Could you check a few things on this model? Use its own coordinates, in mm. Face numbers are marked on the shaded views. Give positions to 0.01 mm unless a question says otherwise; leave off trailing zeros. Loops run counter-clockwise (first coordinate to the right, second up) from the corner with the lowest first, then second, coordinate; pieces in that order, holes last. Notation, with made-up numbers: M 80.5,25.5 L 133.5,25.5 A31 cw 133.5,56.5 Z; hole C 2,74.5 d6. An arc over 180 degrees is marked long. Write each question's results on one line, items separated by ' | '. Start each with the question number.
from build123d import *

# Parameters (mm, degrees)
SKETCH1_W               = 10
SKETCH1_H               = 10
BOSS_EXTRUDE1_DEPTH     = 85
SKETCH2_W               = 10
SKETCH2_H               = 8.2
CUT_EXTRUDE1_DEPTH      = 2.5
CUT_EXTRUDE2_DEPTH      = 86.914201387
CUT_EXTRUDE3_DEPTH      = 2.5
CUT_EXTRUDE3_DEPTH_BACK = 86.914201387
SKETCH4_R               = 1.5
SKETCH5_R               = 1.65
CUT_EXTRUDE4_DEPTH      = 87.168439698


with BuildPart() as part:
    # Sketch1 → Boss-Extrude1 (new body)
    with BuildSketch(Plane(origin=(0, 0, 0), x_dir=(1, 0, 0), z_dir=(0, 1, 0))):
        with Locations((5, 5)):
            Rectangle(SKETCH1_W, SKETCH1_H)
    extrude(amount=BOSS_EXTRUDE1_DEPTH)

    # Sketch2 → Cut-Extrude1 (cut)
    with BuildSketch(Plane(origin=(0, 0, -10), x_dir=(-1, 0, 0), z_dir=(0, 0, -1))):
        with Locations((-5, 65)):
            Rectangle(SKETCH2_W, SKETCH2_H)
    extrude(amount=-CUT_EXTRUDE1_DEPTH, mode=Mode.SUBTRACT)

    # Sketch3 → Cut-Extrude2 (cut, through all)
    with BuildSketch(Plane(origin=(0, 0, -7.5), x_dir=(-1, 0, 0), z_dir=(0, 0, -1))):
        with BuildLine():
            ThreePointArc((-6.75, 65), (-5, 63.25), (-3.25, 65))
            Line((-3.25, 65), (-6.75, 65))
        make_face()
        with BuildLine():
            Line((-6.75, 65), (-3.25, 65))
            ThreePointArc((-3.25, 65), (-5, 66.75), (-6.75, 65))
        make_face()
    extrude(amount=-CUT_EXTRUDE2_DEPTH, mode=Mode.SUBTRACT)

    # Sketch4 → Cut-Extrude3 (cut, two sides: drawn at the far end of the back side and taken through both)
    with BuildSketch(Plane(origin=(0, 0, -7.5), x_dir=(-1, 0, 0), z_dir=(0, 0, -1)).offset(-CUT_EXTRUDE3_DEPTH_BACK)):
        with Locations((-5, 78.856)):
            Circle(SKETCH4_R)
        with Locations((-5, 51.144)):
            Circle(SKETCH4_R)
    extrude(amount=CUT_EXTRUDE3_DEPTH + CUT_EXTRUDE3_DEPTH_BACK, mode=Mode.SUBTRACT)

    # Sketch5 → Cut-Extrude4 (cut, through all)
    with BuildSketch(Plane.XY):
        with Locations((5, 5)):
            Circle(SKETCH5_R)
    extrude(amount=-CUT_EXTRUDE4_DEPTH, mode=Mode.SUBTRACT)


solid = part.part
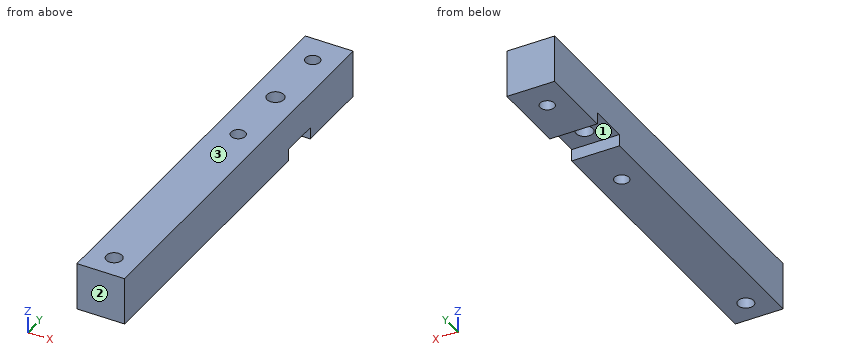
1) If we section it at D-D on z = -1.25: Write out the boundary of the cut face in (x, y).
2) Thinking about a two-plate mould opening in Y: for the marked faces 1, 2 and 3, which applies, pulls with the +Y half, pulls with the -Y half, needs draft (parallel to the pull), parting line crosses it, or undercut?
3) I'm going to push a flat-ended pin straight in: P1, Ø2, axis at x = 5, y = 65, coming from the -Z side. Where does the tip first touch, or does it pass through?
4) If we section it at B-B on x = 5: Write out the boundary of the cut face in (y, z).
5) Please list where these lines run through material, in increasing order: line 1 (Y direction, x = 5, z = -2.25); line 2 (X direction, y = 65, z = -4.25); line 3 (Z direction, x = 6.75, y = 64). Write a range as from..to.
6) If we section it at A-A on y = 65: Write out the boundary of the cut face in (x, z).
7) If we section it at C-C on y = 5: Write out the boundary of the cut face in (x, z), plus the area to 3 significant figures.
Calculated:
1) outline: M 0,0 L 10,0 L 10,85 L 0,85 Z; hole C 5,65 d3.5; hole C 5,5 d3.3; hole C 5,51.14 d3; hole C 5,78.86 d3
2) face 1: undercut | face 2: pulls with the -Y half | face 3: needs draft
3) P1: passes through
4) outline: M 0,-10 L 3.35,-10 L 3.35,0 L 0,0 Z; M 6.65,-10 L 49.64,-10 L 49.64,0 L 6.65,0 Z; M 52.64,-10 L 60.9,-10 L 60.9,-7.5 L 63.25,-7.5 L 63.25,0 L 52.64,0 Z; M 66.75,-7.5 L 69.1,-7.5 L 69.1,-10 L 77.36,-10 L 77.36,0 L 66.75,0 Z; M 80.36,-10 L 85,-10 L 85,0 L 80.36,0 Z
5) line 1: y = 0..3.35, 6.65..49.64, 52.64..63.25, 66.75..77.36, 80.36..85 | line 2: x = 0..3.25, 6.75..10 | line 3: z = -7.5..0
6) outline: M 0,-7.5 L 3.25,-7.5 L 3.25,0 L 0,0 Z; M 6.75,-7.5 L 10,-7.5 L 10,0 L 6.75,0 Z
7) outline: M 0,-10 L 3.35,-10 L 3.35,0 L 0,0 Z; M 6.65,-10 L 10,-10 L 10,0 L 6.65,0 Z | area: 67.0 mm2
